Read the model definition and answer for the solid it produces. Units are mm, in the model's axes. Coordinates: 2 decimals unless noted, no trailing zeros. Order: outer loops, then holes, each group sorted by start corner. A loop starts at its lowest first (then second) coordinate and runs counter-clockwise, first axis right, second up.
Autodesk Inventor part; units mm, degrees
ref_plane "dia1_XY" through (0, 2.3749, 0) normal (1, 0, 0) x (0, 0, -1)
ref_plane "dia1_YZ" through (0, 2.3749, 0) normal (0, 0, -1) x (0, 1, 0)
ref_plane "dia1_ZX" through (0, 2.3749, 0) normal (0, 1, 0) x (1, 0, 0)
sketch "Sketch_1" plane through (0, 0, 0) normal (0, 0, 1) x (1, 0, 0)
  line L0 (100.3808, 0) -> (0, 0)
  line L1 (0, 0) -> (0, 2.3749)
  line L2 (0, 2.3749) -> (68.2752, 2.3749)
  line L3 (68.2752, 2.3749) -> (68.2752, 5.6197)
  line L4 (68.2752, 5.6197) -> (100.3808, 5.6197)
  line L5 (100.3808, 5.6197) -> (100.3808, 0)
  line L6 (100.3808, 0) -> (0, 0)
revolve "Revolution1" add sketch "Sketch_1" angle 360 about axis through (100.3808, 0, 0) along (1, 0, 0)
sketch "Sketch_3" plane through (0, 0, 0) normal (0, 0, 1) x (1, 0, 0)
  line L0 (0, 0) -> (-12.7, 0)
  line L1 (-12.7, 0) -> (-12.7, 1.9406)
  line L2 (-12.7, 1.9406) -> (-12.2276, 2.413)
  line L3 (-12.2276, 2.413) -> (0, 2.413)
  line L4 (0, 2.413) -> (0, 0)
  line L5 (0, 0) -> (-12.7, 0)
revolve "Revolution2" add sketch "Sketch_3" angle 360 about axis through (0, 0, 0) along (1, 0, 0)
thread "Thread1"
sketch "Sketch_30" plane through (0, 0, 0) normal (0, 0, 1) x (1, 0, 0)
  line L0 (0, 0) -> (-0.254, 0)
  line L1 (-0.254, 2.159) -> (0, 2.159)
  line L2 (0, 2.159) -> (0, 2.667)
  line L3 (0, 2.667) -> (-0.254, 2.667)
  line L4 (-0.254, 2.667) -> (-0.254, 2.159)
revolve "Revolution3" cut sketch "Sketch_30" angle 360 about axis through (0, 0, 0) along (1, 0, 0)
ref_plane "dia1_XY" through (0, 2.3749, 0) normal (1, 0, 0) x (0, 0, -1)
ref_plane "dia1_YZ" through (0, 2.3749, 0) normal (0, 0, -1) x (0, 1, 0)
ref_plane "dia1_ZX" through (0, 2.3749, 0) normal (0, 1, 0) x (1, 0, 0)
ref_plane "dia12_XY" through (0, 0, 6.1468) normal (1, 0, 0) x (0, 0, -1)
ref_plane "dia12_YZ" through (0, 0, 6.1468) normal (0, 0, -1) x (0, 1, 0)
ref_plane "dia12_ZX" through (0, 0, 6.1468) normal (0, 1, 0) x (1, 0, 0)
ref_plane "dia2_XY" through (0, -2.3749, 0) normal (1, 0, 0) x (0, 0, -1)
ref_plane "dia2_YZ" through (0, -2.3749, 0) normal (0, 0, -1) x (0, 1, 0)
ref_plane "dia2_ZX" through (0, -2.3749, 0) normal (0, 1, 0) x (1, 0, 0)
ref_plane "dia22_XY" through (0, 0, -6.1468) normal (1, 0, 0) x (0, 0, -1)
ref_plane "dia22_YZ" through (0, 0, -6.1468) normal (0, 0, -1) x (0, 1, 0)
ref_plane "dia22_ZX" through (0, 0, -6.1468) normal (0, 1, 0) x (1, 0, 0)
ref_plane "rl1_XY" through (-12.7, 0, 0) normal (1, 0, 0) x (0, 0, -1)
ref_plane "rl1_YZ" through (-12.7, 0, 0) normal (0, 0, -1) x (0, 1, 0)
ref_plane "rl1_ZX" through (-12.7, 0, 0) normal (0, 1, 0) x (1, 0, 0)
ref_plane "rl2_XY" through (0, 0, 0) normal (1, 0, 0) x (0, 0, -1)
ref_plane "rl2_YZ" through (0, 0, 0) normal (0, 0, -1) x (0, 1, 0)
ref_plane "rl2_ZX" through (0, 0, 0) normal (0, 1, 0) x (1, 0, 0)
ref_plane "rod_cp_XY" through (0, 0, 0) normal (1, 0, 0) x (0, 0, -1)
ref_plane "rod_cp_YZ" through (0, 0, 0) normal (0, 0, -1) x (0, 1, 0)
ref_plane "rod_cp_ZX" through (0, 0, 0) normal (0, 1, 0) x (1, 0, 0)
ref_plane "thd1_XY" through (-12.7, 2.413, 0) normal (1, 0, 0) x (0, 0, -1)
ref_plane "thd1_YZ" through (-12.7, 2.413, 0) normal (0, 0, -1) x (0, 1, 0)
ref_plane "thd1_ZX" through (-12.7, 2.413, 0) normal (0, 1, 0) x (1, 0, 0)
ref_plane "thd2_XY" through (-12.7, -2.413, 0) normal (1, 0, 0) x (0, 0, -1)
ref_plane "thd2_YZ" through (-12.7, -2.413, 0) normal (0, 0, -1) x (0, 1, 0)
ref_plane "thd2_ZX" through (-12.7, -2.413, 0) normal (0, 1, 0) x (1, 0, 0)
ref_plane "to_rod_clevis_XY" through (-12.7, 0, 0) normal (1, 0, 0) x (0, 0, -1)
ref_plane "to_rod_clevis_YZ" through (-12.7, 0, 0) normal (0, 0, -1) x (0, 1, 0)
ref_plane "to_rod_clevis_ZX" through (-12.7, 0, 0) normal (0, 1, 0) x (1, 0, 0)
properties part number "M-011-BT1EE110_rod"
1) Straight lines are drawn through the part: line 1 (X direction, y = -2, z = -2.75); line 2 (Y direction, x = 84, z = -0.5); line 3 (Y direction, x = 68, z = -0.25). For each, find the intervals that lie inside material, in ascending order.
A:
line 1: x = 68.28 to 100.38
line 2: y = -5.6 to 5.6
line 3: y = -2.36 to 2.36
2) A cutting plane is placed at D-D, the plane x = -5. Determine the outline of the cut face in (y, z), and give its area (3 significant figures).
A:
outline: circle Ø4.83 at (0, 0)
area: 18.3 mm2
3) A cutting plane is placed at A-A, the plane y = 0. Determine the outline of the cut face in (x, z), and give its area (3 significant figures).
A:
outline: (-12.7, -1.94) - (-12.23, -2.41) - (-0.25, -2.41) - (-0.25, -2.16) - (0, -2.16) - (0, -2.37) - (68.28, -2.37) - (68.28, -5.62) - (100.38, -5.62) - (100.38, 5.62) - (68.28, 5.62) - (68.28, 2.37) - (0, 2.37) - (0, 2.16) - (-0.25, 2.16) - (-0.25, 2.41) - (-12.23, 2.41) - (-12.7, 1.94) - close
area: 746 mm2
4) A cutting plane is placed at C-C, the plane x = 48. Determine the outline of the cut face in (y, z).
A:
outline: circle Ø4.75 at (0, 0)
5) Determine the mould class of faces 1 (the cylindrical face through (84.553, -1.218, -5.486)), 2 (the flat face through (-12.7, 0, 0)), 3 (the flat face through (100.381, 0, 0)) for opening direction X: pulls with the +X half, pulls with the -X half, needs draft (parallel to the pull), parting line crosses it, or undercut.
A:
face 1: needs draft
face 2: pulls with the -X half
face 3: pulls with the +X half
6) Flat-ended cylindrical pins translate along their axes: pin 1 Ø6 at (x, z) = (41, -3.5) entering from -Y; pin 2 Ø2 at (x, z) = (8, 2) entering from +Y; pin 3 Ø5 at (x, y) = (84, 4) entering from +Z. Find the tip coordinate at first contact, or state that the pin passes through.
A:
pin 1: stops at y = -2.32
pin 2: stops at y = 2.15
pin 3: stops at z = 5.42
